Autodesk Inventor part; units mm, degrees
ref_plane "YZ Plane" through (0, 0, 0) normal (1, 0, 0) x (0, 1, 0)
ref_plane "XZ Plane" through (0, 0, 0) normal (0, 1, 0) x (-1, 0, 0)
ref_plane "XY Plane" through (0, 0, 0) normal (0, 0, 1) x (1, 0, 0)
sketch "Sketch1" plane through (0, 0, 0) normal (0, 0, 1) x (1, 0, 0)
  line L0 (0, 0) -> (28, 0)
  line L1 (28, 0) -> (28, 18)
  line L2 (28, 18) -> (0, 18)
  line L3 (0, 18) -> (0, 0)
  dimension "d0" = 28
  dimension "d1" = 18
  dimension "d2" = 28
extrude "Extrusion1" add sketch "Sketch1" along normal blind 1
sketch "Sketch2" plane through (0, 0, 1) normal (0, 0, 1) x (1, 0, 0)
  line L0 (21.3992, 11.8771) -> (21.3992, 6.4359)
  line L1 (21.3992, 6.4359) -> (12.5353, 6.4359)
  line L2 (12.5353, 6.4359) -> (12.5353, 11.8771)
  line L3 (12.5353, 11.8771) -> (21.3992, 11.8771)
  line L4 (3.7591, 12.6669) -> (3.7591, 10.8901)
  line L5 (3.7591, 10.8901) -> (4.997, 10.8901)
  line L6 (4.997, 10.8901) -> (4.997, 12.6669)
  line L7 (4.997, 12.6669) -> (3.7591, 12.6669)
  line L8 (3.4697, 8.4681) -> (7.5353, 8.4681)
  line L9 (7.5353, 8.4681) -> (7.5353, 4.1843)
  line L10 (7.5353, 4.1843) -> (3.4697, 4.1843)
  line L11 (3.4697, 4.1843) -> (3.4697, 8.4681)
  point P0 (0, 0)
extrude "Extrusion2" add sketch "Sketch2" along normal blind 1
sketch "Sketch3" plane through (28, 0, 0) normal (1, 0, 0) x (0, 0, -1)
  line L0 (-1, 6.4359) -> (-1, 11.8771)
  line L1 (-1, 9.1565) -> (-3.5, 9.1565)
  line L2 (-3.5, 9.1565) -> (-3.5, 13.1565)
  line L3 (-3.5, 13.1565) -> (-3.5, 5.1565)
  line L4 (-2, 8.4681) -> (-2, 4.1843)
  line L5 (-2, 11.8771) -> (-2, 6.4359)
  line L6 (-2, 9.1565) -> (-2, 6.3262)
  arc A0 (-3.5, 5.1565) -> (-1, 6.4359) centre (-3.4729, 8.1858) ccw
  arc A1 (-1, 11.8771) -> (-3.5, 13.1565) centre (-3.6026, 9.8737) ccw
  line L7 (-1, 6.4359) -> (-1, 11.8771)
  point P0 (0, 0)
  dimension "d7" = 2.5
  dimension "d8" = 4
  dimension "d9" = 8
extrude "Extrusion3" add sketch "Sketch3" along normal blind 1
sketch "Sketch4" plane through (28, 0, 0) normal (-1, 0, 0) x (0, 0, 1)
  arc A0 (3.5, 13.1565) -> (1, 11.8771) centre (3.6026, 9.8737) ccw
  line L0 (1, 6.4359) -> (1, 11.8771)
  arc A1 (1, 6.4359) -> (3.5, 5.1565) centre (3.4729, 8.1858) ccw
  line L1 (3.5, 13.1565) -> (3.5, 5.1565)
  point P0 (0, 0)
extrude "Extrusion4" add sketch "Sketch4" along normal blind 4
properties part number "Regulador"
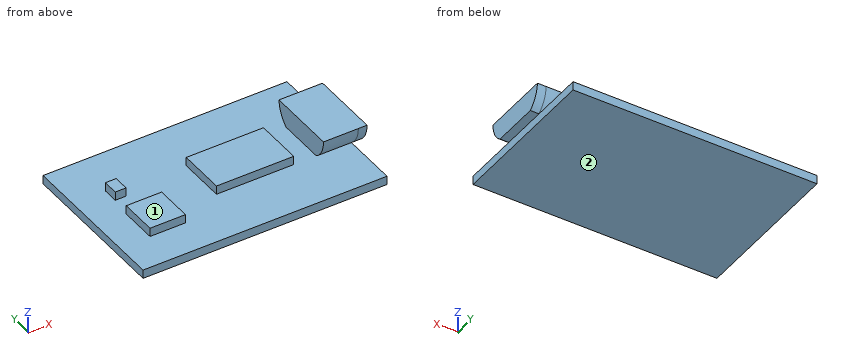
Could you check a few things on this model? Use its own coordinates, in mm. Face numbers are marked on the shaded views. A direction names the side the tool comes from. Coordinates: 2 decimals unless noted, no trailing zeros. Order: outer loops, then holes, each group sorted by start corner. A loop starts at its lowest first (then second) coordinate and runs counter-clockwise, first axis right, second up. Notation, with made-up numbers: M 4,33 L 49,33 A25 ccw 49,68 Z; hole C 70.5,72 d6. An arc over 180 degrees is marked long. Use one line per item in the form item = value. Start each with the question number.
1. Please list where these lines run through material, in increasing order: line 1 (X direction, y = 17, z = 0.5); line 2 (X direction, y = 13, z = 2.8); line 3 (Z direction, x = 10.25, y = 5.5).
2. Suppose I cut it at A-A on x = 19.25. Write out the boundary of the cut face in (y, z), then the cut area to 3 significant figures.
3. Suppose I cut it at B-B on y = 10. Write out the boundary of the cut face in (x, z), then the cut area to 3 significant figures.
4. For pin 1 (1 mm diameter, centred on x = 4, y = 12, fed in from +Z); pin 2 (1.3 mm diameter, centred on y = 11, z = 2.5, fed in from -X); pin 3 (0.5 mm diameter, centred on x = 5.5, z = 1.5, fed in from -Y), each with a flat end and sliding along its axis, tell me the tip position at first contact or that it passes through.
5. On a 3-axis mill with a long thin cutter (end or side, diameter ignored), from which of +Z, -Z, +X, -X, +Y, -Y can I reach the whole of each face in a straight line? I mean the marked faces 1 and 2. Say none if no direction works.
6. Suppose I cut it at C-C on z = 1.5. Count the separate pieces of the cut face and the enclosed holes in it, then the cut area to 3 significant figures.
Geometry says:
q1.line_1 = 0 to 28
q1.line_2 = 24 to 29
q1.line_3 = 0 to 1
q2.outline = M 0,0 L 18,0 L 18,1 L 11.88,1 L 11.88,2 L 6.44,2 L 6.44,1 L 0,1 Z
q2.area = 23.4 mm^2
q3.outline = M 0,0 L 28,0 L 28,1 L 29,1 L 29,3.5 L 24,3.5 L 24,1 L 21.4,1 L 21.4,2 L 12.54,2 L 12.54,1 L 0,1 Z
q3.area = 49.4 mm^2
q4.pin_1 = 2
q4.pin_2 = 3.76
q4.pin_3 = 4.18
q5.face_1 = +Z, -X, +Y, -Y
q5.face_2 = -Z, +X, -X, +Y, -Y
q6.separate_pieces = 4
q6.enclosed_holes = 0
q6.area = 100 mm^2
